The model under review builds one solid part; all positions refer to its coordinate system, in mm. Round coordinates to 2 decimals unless told otherwise and drop trailing zeros. Write each loop counter-clockwise with the first axis right and the second up, starting at its lowest first coordinate (ties: lowest second). Pieces come first, ordered by that corner, then holes.
Item 1: Add section C-C (y = -80). Give the boundary of the cut face in (x, z), plus the area to 3 significant figures.
Item 2: To check wall thickness, follow L1, parallel to Y at x = 0, z = -1.75; L2, parallel to Y at x = -9, z = -1.95; L3, parallel to Y at x = -4.5, z = -2. State the ranges of each line that lie inside material, in increasing order.
Item 3: Add section B-B (z = -0.9). State how many separate pieces and enclosed holes the cut face has, plus the area to 3 significant figures.
Item 4: Add section A-A (y = 0). Give the boundary of the cut face in (x, z), plus the area to 3 significant figures.
Autodesk Inventor part; units mm, degrees
ref_plane "YZ Plane" through (0, 0, 0) normal (1, 0, 0) x (0, 1, 0)
ref_plane "XZ Plane" through (0, 0, 0) normal (0, 1, 0) x (-1, 0, 0)
ref_plane "XY Plane" through (0, 0, 0) normal (0, 0, 1) x (1, 0, 0)
sketch "スケッチ1" plane through (0, 0, 0) normal (0, 0, 1) x (1, 0, 0)
  circle A0 centre (0, 0) radius 21.2
  circle A1 centre (0, 0) radius 7.5
  circle A2 centre (0, 0) radius 30
  circle A3 centre (20.819222, -21.6) radius 22.5
  circle A4 centre (20.819222, -21.6) radius 14
  circle A5 centre (20.819222, -21.6) radius 62
  circle A6 centre (0, -80) radius 48
  circle A7 centre (0, -80) radius 50
  circle A8 centre (20.819222, -21.6) radius 4
  circle A9 centre (0, -80) radius 5
  dimension "d2" = 60
  dimension "d4" = 124
  dimension "d0" = 42.4
  dimension "d1" = 15
  dimension "d3" = 28
  dimension "d5" = 100
  dimension "d23" = 8
  dimension "d24" = 10
sketch "スケッチ2" plane through (0, 0, 0) normal (0, 0, 1) x (1, 0, 0)
  line L0 (0, 0) -> (24.501973, 0) construction
  line L1 (0, 0) -> (12.5, 0) construction
  line L2 (0, 0) -> (10.253048, 10.253048)
  line L3 (0, 0) -> (14.5, 0) construction
  line L4 (10.253048, 10.253048) -> (-10.253048, -10.253048)
  circle A0 centre (10.253048, 10.253048) radius 2
  circle A1 centre (-10.253048, -10.253048) radius 2
  circle A2 centre (0, 0) radius 7.5
  line L5 (0, 0) -> (28.190779, 10.260604)
  line L6 (0, 0) -> (30, 0) construction
  line L7 (0, 0) -> (-28.190779, 10.260604)
  line L8 (0, 0) -> (30, 0) construction
  circle A3 centre (-28.190779, 10.260604) radius 2.5
  line L9 (0, 0) -> (0, 30)
  circle A4 centre (0, 30) radius 2.5
  circle A5 centre (28.190779, 10.260604) radius 2.5
  dimension "d9" = 14.5
  dimension "d10" = 45
  dimension "d11" = 29
  dimension "d12" = 4
  dimension "d13" = 4
  dimension "d14" = 15
  dimension "d15" = 30
  dimension "d16" = 20
  dimension "d17" = 30
  dimension "d18" = 160
  dimension "d19" = 5
  dimension "d20" = 30
  dimension "d21" = 5
  dimension "d22" = 5
sketch "スケッチ3" plane through (0, 0, 0) normal (0, 0, 1) x (1, 0, 0)
  line L0 (60, -99.343647) -> (-60, -99.343647)
  line L1 (-60, -99.343647) -> (-60, 99.343647)
  line L2 (-60, 99.343647) -> (60, 99.343647)
  line L3 (60, 99.343647) -> (60, -99.343647)
  line L4 (60, -99.343647) -> (-60, 99.343647) construction
  line L5 (-60, -99.343647) -> (60, 99.343647) construction
  point P0 (0, 0)
  dimension "d25" = 120
extrude "押し出し1" add sketch "スケッチ3" against normal blind 3
extrude "押し出し2" cut sketch "スケッチ2" against normal blind 3
extrude "押し出し3" cut sketch "スケッチ1" against normal blind 3 contours A8 A2 | A2 A8 | A9 A5 | A5 A9
sketch "スケッチ4" plane through (0, 0, 0) normal (0, 0, 1) x (1, 0, 0)
  line L0 (0, 45.071117) -> (68.359536, 45.071117)
  line L1 (68.359536, 45.071117) -> (-74.382402, 45.071117)
  line L2 (-74.382402, 45.071117) -> (108.165644, 45.071117)
  line L3 (108.165644, 45.071117) -> (108.165644, 129.415375)
  line L4 (108.165644, 129.415375) -> (-74.382402, 129.415375)
  line L5 (-74.382402, 129.415375) -> (-74.382402, 45.071117)
  point P0 (0, 0)
extrude "押し出し4" cut sketch "スケッチ4" against normal blind 10
fillet "フィレット1" radius 4 4 edges at (-60, 45.0711, -1.5) (60, 45.0711, -1.5) (-60, -99.3436, -1.5) (60, -99.3436, -1.5)
sketch "スケッチ5" plane through (0, 0, 0) normal (0, 0, 1) x (1, 0, 0)
  circle A0 centre (0, -80) radius 5
  circle A1 centre (0, -80) radius 11
  point P0 (0, 0)
  dimension "d35" = 22
extrude "押し出し5" cut sketch "スケッチ5" against normal blind 10
sketch "スケッチ6" plane through (0, 0, 0) normal (0, 0, 1) x (1, 0, 0)
  circle A0 centre (20.819222, -21.6) radius 4
  circle A1 centre (20.819222, -21.6) radius 7
  point P0 (0, 0)
  dimension "d38" = 14
extrude "押し出し6" cut sketch "スケッチ6" against normal through all
properties part number "板"
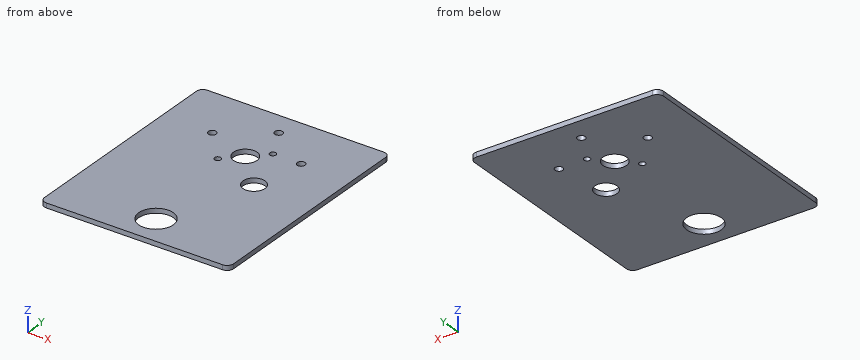
Numbers:
1. outline: (-60, -3) - (-11, -3) - (-11, 0) - (-60, 0) - close; (11, -3) - (60, -3) - (60, 0) - (11, 0) - close
1. area: 294 mm2
2. L1: y = -99.34 to -91, -69 to -7.5, 7.5 to 27.5, 32.5 to 45.07
2. L2: y = -99.34 to -86.32, -73.68 to -11.81, -8.69 to 45.07
2. L3: y = -99.34 to -90.04, -69.96 to -6, 6 to 45.07
3. separate pieces: 1
3. enclosed holes: 8
3. area: 16,500 mm2
4. outline: (-60, -3) - (-7.5, -3) - (-7.5, 0) - (-60, 0) - close; (7.5, -3) - (60, -3) - (60, 0) - (7.5, 0) - close
4. area: 315 mm2
